For this review, take the finished solid that the model builds, in its own axes (mm). A direction names the side the tool comes from. Give positions to 0.01 mm unless a question says otherwise; leave off trailing zeros. Order: outer loops, then holes, each group sorted by start corner. A loop starts at its lowest first (then second) coordinate and runs counter-clockwise, first axis right, second up. Notation, with made-up numbers: (63, 1.5) - (106, 1.5) arc R30 cw to (106, 40.5) - close; hole circle Ø8 at (-22, 32). An arc over 180 degrees is marked (long way). Answer as a JSON object with one key per item and string values. Group by question number.
from build123d import *

# Parameters (mm, degrees)
F0_W     = 63.5
F0_H     = 63.5
F1_DEPTH = 12.7
F2_W     = 63.5
F2_H     = 12.7
F3_DEPTH = 50.8
F4_W     = 12.7
F4_H     = 50.8
F5_DEPTH = 50.8
F6_W     = 12.7
F6_H     = 12.7
F7_DEPTH = 25.4


with BuildPart() as f1:
    # F0 (on Top) → F1 (new body)
    with BuildSketch(Plane.XY):
        with Locations((31.75, -31.75)):
            Rectangle(F0_W, F0_H)
    extrude(amount=F1_DEPTH)

    # F2 (on face) → F3 (join)
    with BuildSketch(Plane.XY.offset(12.7)):
        with Locations((31.75, -6.35)):
            Rectangle(F2_W, F2_H)
    extrude(amount=F3_DEPTH)

    # F4 (on face) → F5 (join)
    with BuildSketch(Plane.XY.offset(12.7)):
        with Locations((6.35, -38.1)):
            Rectangle(F4_W, F4_H)
    extrude(amount=F5_DEPTH)

    # F6 (on face) → F7 (cut)
    with BuildSketch(Plane.XY.offset(12.7)):
        with Locations((57.15, -57.15)):
            Rectangle(F6_W, F6_H)
    extrude(amount=-F7_DEPTH, mode=Mode.SUBTRACT)


solid = f1.part
1) Consider section B-B (x = 20.5). Give the boundary of the cut face in (y, z).
2) For pin 1 (10 mm diameter, centred on y = -31, z = 22.5, fed in from -X); pin 2 (6 mm diameter, centred on y = -50.5, z = 22, fed in from +X); pin 3 (6.5 mm diameter, centred on x = 57.5, z = 6, fed in from -Y); pin 4 (1.5 mm diameter, centred on x = 53.5, y = -51, fed in from +Z), all flat-tipped, find the tip position at first contact; note any pin that passes through.
3) Consider section A-A (y = -52.5). Give the boundary of the cut face in (x, z), plus the area to 3 significant figures.
4) For faces 1 (the face through (50.8, -57, 6)), 2 (the face through (31, -31, 0)), 3 (the face through (12.7, -38, 38)), list the 3-axis set-ups (+Z, -Z, +X, -X, +Y, -Y) from which the entire face can be reached by the end or side of a thin tool; tool diameter is ignored.
5) For line 1 (Z direction, x = 59.5, y = -31); line 2 (Y direction, x = 22.5, z = 58.5), list the stretches that pass through material, from the lowest coordinate up.
Result set:
{
 "1": {"outline": "(-63.5, 0) - (0, 0) - (0, 63.5) - (-12.7, 63.5) - (-12.7, 12.7) - (-63.5, 12.7) - close"},
 "2": {"pin 1": "stops at x = 0", "pin 2": "stops at x = 12.7", "pin 3": "stops at y = -50.8", "pin 4": "stops at z = 12.7"},
 "3": {"outline": "(0, 0) - (50.8, 0) - (50.8, 12.7) - (12.7, 12.7) - (12.7, 63.5) - (0, 63.5) - close", "area": "1,290 mm2"},
 "4": {"face 1": "+Z, -Z, +X, -Y", "face 2": "-Z, +X, -X, +Y, -Y", "face 3": "+Z, +X, -Y"},
 "5": {"line 1": "z = 0 to 12.7", "line 2": "y = -12.7 to 0"}
}
